from build123d import *

# Parameters (mm, degrees)
SKICA2_W                  = 130
SKICA2_H                  = 50
P_IDAT_VYSUNUT_M1_DEPTH   = 10
P_IDAT_START              = -10
SKICA2_7_W                = 122
SKICA2_7_H                = 12
P_IDAT_VYSUNUT_M3_DEPTH   = 7
SKICA2_8_W                = 40
SKICA2_8_H                = 18
P_IDAT_VYSUNUT_M4_DEPTH   = 2.2
SKICA3_W                  = 5.6
SKICA3_H                  = 13.2
ODEBRAT_VYSUNUT_M12_DEPTH = 11
SKICA4_W                  = 126
SKICA4_H                  = 46
SKICA4_W_2                = 124
SKICA4_H_2                = 44
P_IDAT_VYSUNUT_M5_DEPTH   = 5
ZAOBLIT1_R                = 2


with BuildPart() as part:
    # Skica2 → Přidat vysunutím1 (new body)
    with BuildSketch(Plane.XY):
        with Locations((-0.5, 0)):
            Rectangle(SKICA2_W, SKICA2_H)
        Polygon((-62.5, -15), (-62.5, -3), (-62.5, 15), (-22.5, 15), (-22.5, -3), (59.5, -3), (59.5, -15), align=None, mode=Mode.SUBTRACT)
    extrude(amount=-P_IDAT_VYSUNUT_M1_DEPTH)

    # Skica2<7> → Přidat vysunutím3 (add)
    with BuildSketch(Plane.XY.offset(P_IDAT_START)):
        with Locations((-1.5, -9)):
            Rectangle(SKICA2_7_W, SKICA2_7_H)
    extrude(amount=P_IDAT_VYSUNUT_M3_DEPTH)

    # Skica2<8> → Přidat vysunutím4 (add)
    with BuildSketch(Plane.XY.offset(P_IDAT_START)):
        with Locations((-42.5, 6)):
            Rectangle(SKICA2_8_W, SKICA2_8_H)
    extrude(amount=P_IDAT_VYSUNUT_M4_DEPTH)

    # Skica3 → Odebrat vysunutím12 (cut)
    with BuildSketch(Plane.ZY.offset(65.5)):
        with Locations((-5, 5.4)):
            Rectangle(SKICA3_W, SKICA3_H)
    extrude(amount=-ODEBRAT_VYSUNUT_M12_DEPTH, mode=Mode.SUBTRACT)

    # Skica4 → Přidat vysunutím5 (add)
    with BuildSketch(Plane.XY):
        with Locations((-0.5, 0)):
            Rectangle(SKICA4_W, SKICA4_H)
        with Locations((-0.5, 0)):
            Rectangle(SKICA4_W_2, SKICA4_H_2, mode=Mode.SUBTRACT)
    extrude(amount=P_IDAT_VYSUNUT_M5_DEPTH)

    # Zaoblit1
    zaoblit1_edges = [part.edges().sort_by_distance(p)[0] for p in [
        (-65.5, -25, -5),
        (-65.5, 25, -5),
        (64.5, 25, -5),
        (64.5, -25, -5),
    ]]
    fillet(zaoblit1_edges, radius=ZAOBLIT1_R)


solid = part.part
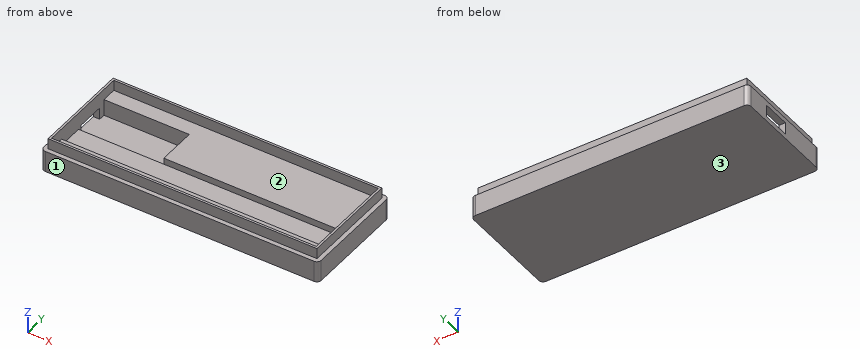
Could you check a few things on this model? Use its own coordinates, in mm. Face numbers are marked on the shaded views. Give positions to 0.01 mm unless a question says otherwise; leave off trailing zeros. Loops run counter-clockwise (first coordinate to the right, second up) from the corner with the lowest first, then second, coordinate; pieces in that order, holes last. Notation, with made-up numbers: M 34.25,-2.75 L 57.25,-2.75 A29 ccw 57.25,29.25 Z; hole C 21,-21 d5. An arc over 180 degrees is marked long. Answer as a JSON object with one key per item and string values.
Q1. Suppose I cut it at A-A, the plane y = 10.5. List the corners of the cut face in (x, z) for me.
Values found:
{"outline": "M -65.5,-10 L 64.5,-10 L 64.5,0 L 62.5,0 L 62.5,5 L 61.5,5 L 61.5,0 L -22.5,0 L -22.5,-7.8 L -65.5,-7.8 Z; M -65.5,-2.2 L -62.5,-2.2 L -62.5,5 L -63.5,5 L -63.5,0 L -65.5,0 Z"}
Q2. For P1, Ø2, axis at x = -32.5, z = 0.5, coming from the +Y side; P2, Ø2.5, axis at x = 15.5, z = 1.5, coming from the -Y side; P3, Ø5.5, axis at y = 1.5, z = 3, coming from the +X side; P4, Ø10, axis at x = 21.5, y = -16.5, coming from the +Z side, each with a flat end and sliding along its axis, tell me the tip position at first contact or that it passes through.
Values found:
{"P1": "stops at y = 25", "P2": "stops at y = -23", "P3": "stops at x = 62.5", "P4": "stops at z = 0"}
Q3. Suppose I cut it at D-D, the plane z = -6. List the corners of the cut face in (x, y) for me.
Values found:
{"outline": "M -65.5,-23 A2 ccw -63.5,-25 L 62.5,-25 A2 ccw 64.5,-23 L 64.5,23 A2 ccw 62.5,25 L -63.5,25 A2 ccw -65.5,23 L -65.5,12 L -62.5,12 L -62.5,15 L -22.5,15 L -22.5,-3 L -62.5,-3 L -62.5,-1.2 L -65.5,-1.2 Z"}
Q4. Suppose I cut it at C-C, the plane x = 46. List the corners of the cut face in (y, z) for me.
Values found:
{"outline": "M -25,-10 L 25,-10 L 25,0 L 23,0 L 23,5 L 22,5 L 22,0 L -3,0 L -3,-3 L -15,-3 L -15,0 L -22,0 L -22,5 L -23,5 L -23,0 L -25,0 Z"}
Q5. Suppose I cut it at B-B, the plane z = 1.5. List the corners of the cut face in (x, y) for me.
Values found:
{"outline": "M -63.5,-23 L 62.5,-23 L 62.5,23 L -63.5,23 Z; hole M -62.5,-22 L 61.5,-22 L 61.5,22 L -62.5,22 Z"}
Q6. If I drill on probe 1 along X at (y, z) = (-11, 4); probe 2 along Y at (x, z) = (-26.5, -6); probe 3 along Y at (x, z) = (-45.5, 2.5), over which ranges is the centre line in solid material (lowest first)? Write a range as [from, to].
Values found:
{"probe 1": "x = [-63.5, -62.5], [61.5, 62.5]", "probe 2": "y = [-25, -3], [15, 25]", "probe 3": "y = [-23, -22], [22, 23]"}
Q7. If we mould it in two halves opening along Y, with no side actions, what happens to the marked faces 1, 2 and 3? For each: pulls with the +Y half, pulls with the -Y half, needs draft (parallel to the pull), parting line crosses it, or undercut.
Values found:
{"face 1": "pulls with the -Y half", "face 2": "undercut", "face 3": "needs draft"}
